```python
from build123d import *

# Parameters (mm, degrees)
BOSS_EXTRUDE1_DEPTH = 0.635
SKETCH2_W           = 5.08
SKETCH2_H           = 2.8575
BOSS_EXTRUDE2_DEPTH = 2.8575
FILLET1_R           = 1.42875
SKETCH3_R           = 0.714375
CUT_EXTRUDE1_DEPTH  = 30


with BuildPart() as part:
    # Sketch1 → Boss-Extrude1 (new body)
    with BuildSketch(Plane(origin=(0, 0, 0), x_dir=(1, 0, 0), z_dir=(0, 1, 0))):
        Polygon((12.849131833, 13.383236071), (7.769131833, 13.383236071), (7.769131833, 10.525736071), (2.689131833, 10.525736071), (2.689131833, -0.745513929), (28.089131833, -0.745513929), (28.089131833, 10.525736071), (23.009131833, 10.525736071), (23.009131833, 13.383236071), (17.929131833, 13.383236071), (17.929131833, 10.525736071), (12.849131833, 10.525736071), align=None)
    extrude(amount=BOSS_EXTRUDE1_DEPTH)

    # Sketch2 → Boss-Extrude2 (add)
    with BuildSketch(Plane(origin=(0, 0.635, 0), x_dir=(1, 0, 0), z_dir=(0, 1, 0))):
        with Locations((10.309131833, 11.954486071)):
            Rectangle(SKETCH2_W, SKETCH2_H)
        with Locations((20.469131833, 11.954486071)):
            Rectangle(SKETCH2_W, SKETCH2_H)
    extrude(amount=-BOSS_EXTRUDE2_DEPTH)

    # Fillet1
    fillet1_edges = [part.edges().sort_by_distance(p)[0] for p in [
        (10.309131833, -2.2225, -10.525736071),
        (20.469131833, -2.2225, -10.525736071),
        (20.469131833, -2.2225, -13.383236071),
        (10.309131833, -2.2225, -13.383236071),
        (10.309131833, 0.635, -13.383236071),
        (20.469131833, 0.635, -13.383236071),
    ]]
    fillet(fillet1_edges, radius=FILLET1_R - 0.0001)  # a hair under: the kernel refuses the full size

    # Sketch3 → Cut-Extrude1 (cut)
    with BuildSketch(Plane(origin=(23.009131833, 0, 0), x_dir=(0, 0, -1), z_dir=(1, 0, 0))):
        with Locations((11.954486071, -0.79375)):
            Circle(SKETCH3_R)
    extrude(amount=-CUT_EXTRUDE1_DEPTH, mode=Mode.SUBTRACT)


solid = part.part
```
Model file for the job. Use its own axes, mm. A direction names the side the tool comes from. Round coordinates to 2 decimals unless told otherwise and drop trailing zeros. Order: outer loops, then holes, each group sorted by start corner. A loop starts at its lowest first (then second) coordinate and runs counter-clockwise, first axis right, second up. Notation, with made-up numbers: M -22,15.5 L 23,15.5 A8 cw 23,24.5 Z; hole C -14.5,-25.5 d4. An arc over 180 degrees is marked long. Use CSV: the item, a comma, the result in double quotes.
Item 1: Saw through at D-D (y = 0.3). List the corners of the cut face in (x, z), plus the area to 3 significant figures.
Worked answers:
outline,"M 2.69,-10.53 L 7.77,-10.53 L 7.77,-12.87 L 12.85,-12.87 L 12.85,-10.53 L 17.93,-10.53 L 17.93,-12.87 L 23.01,-12.87 L 23.01,-10.53 L 28.09,-10.53 L 28.09,0.75 L 2.69,0.75 Z"
area,"310 mm²"
Item 2: Pull direction Z, two halves, no side cores. Call faces 5 (the face through (15, 0, -5)), 6 (the face through (20.434, 0.205, -12.976)), 7 (the face through (10.345, -0.579, -12.636)): released by +Z, released by -Z, zero draft, split by the parting line, or undercut.
Worked answers:
face 5,"zero draft"
face 6,"released by -Z"
face 7,"undercut"
Item 3: Saw through at A-A (y = -1.15). List the corners of the cut face in (x, z), plus the area to 3 significant figures.
Worked answers:
outline,"M 7.77,-13.34 L 12.85,-13.34 L 12.85,-12.57 L 7.77,-12.57 Z; M 7.77,-11.34 L 12.85,-11.34 L 12.85,-10.57 L 7.77,-10.57 Z; M 17.93,-13.34 L 23.01,-13.34 L 23.01,-12.57 L 17.93,-12.57 Z; M 17.93,-11.34 L 23.01,-11.34 L 23.01,-10.57 L 17.93,-10.57 Z"
area,"15.5 mm²"
Item 4: Pin check, flat tips, straight feed: pin 1 (1.4 mm diameter, centred on y = -0.5, z = -12, fed in from -X); pin 2 (0.7 mm diameter, centred on x = 16.5, y = 0.5, fed in from -Z); pin 3 (3 mm diameter, centred on x = 14.5, z = -1.5, fed in from -Y). Stop position of each tip, or through.
Worked answers:
pin 1,"x = 7.77"
pin 2,"z = -10.53"
pin 3,"y = 0"
Item 5: Probe probe 1 along X at (y, z) = (0.1, -11.75); probe 2 along Y at (x, z) = (10.75, -12.5) (1 decimal); probe 3 along Z at (x, y) = (20, -1.2). List the from-to ranges inside material, lowest first.
Worked answers:
probe 1,"7.77 to 12.85, 17.93 to 23.01"
probe 2,"-2.1 to -1.3, -0.3 to 0.5"
probe 3,"-13.32 to -12.54, -11.37 to -10.58"
Item 6: Which spindle directions (+Z, -Z, +X, -X, +Y, -Y) get a long thin tool onto all of the face, cutting with end or side? Do faces 1 (the face through (7.769, 0, -11)), 2 (the face through (20.5, -1.82, -12.95)), 3 (the face through (23.009, 0, -11)), 4 (the face through (17.929, 0, -11)). Say none if no direction does.
Worked answers:
face 1,"-Z, -X, +Y, -Y"
face 2,"-Z, +X, -X, -Y"
face 3,"-Z, +X, +Y, -Y"
face 4,"-Z, +Y, -Y"
Item 7: Saw through at C-C (z = -5). List the corners of the cut face in (x, y) (3 decimals), plus the area to 3 significant figures.
Worked answers:
outline,"M 2.689,0 L 28.089,0 L 28.089,0.635 L 2.689,0.635 Z"
area,"16.1 mm²"
